```python
from build123d import *

# Parameters (mm, degrees)
F1_DEPTH = 101.6
F2_W     = 62.831107527
F2_H     = 56.3771557063
F3_DEPTH = 36.068
F4_W     = 26.6572609544
F4_H     = 13.4982671589
F4_H_2   = 14.6736167371
F5_DEPTH = 108.712
F6_R     = 7.0273260197
F6_R_2   = 6.9955111579
F6_R_3   = 6.6555032816
F6_R_4   = 6.7798018692
F7_DEPTH = 174.752


with BuildPart() as f1:
    # F0 (on Front) → F1 (new body)
    with BuildSketch(Plane.XZ):
        Polygon((-7.4572972953, 38.0593240261), (-75.9830623865, 38.0593240261), (-75.9830623865, -18.1280076504), (0, -18.1280076504), (0, -31.7951962352), (76.0644078255, -31.7951962352), align=None)
    extrude(amount=F1_DEPTH)

    # F2 (on face) → F3 (cut)
    with BuildSketch(Plane.XZ.offset(101.6)):
        with Locations((59.3193974346, -3.606618382)):
            Rectangle(F2_W, F2_H)
    extrude(amount=-F3_DEPTH, mode=Mode.SUBTRACT)

    # F4 (on face) → F5 (cut)
    with BuildSketch(Plane(origin=(-75.9830623865, 0, 0), x_dir=(0, -1, 0), z_dir=(-1, 0, 0))):
        with Locations((50.1333586872, 31.3101904467)):
            Rectangle(F4_W, F4_H)
        with Locations((50.1333586872, 45.3961323947)):
            Rectangle(F4_W, F4_H_2)
    extrude(amount=-F5_DEPTH, mode=Mode.SUBTRACT)

    # F6 (on face) → F7 (cut)
    with BuildSketch(Plane(origin=(-75.9830623865, 0, 0), x_dir=(0, -1, 0), z_dir=(-1, 0, 0))):
        with Locations((51.6176335514, -6.4415424131)):
            Circle(F6_R)
        with Locations((51.6176335514, 13.1108649075)):
            Circle(F6_R_2)
        with Locations((17.7108142525, -6.4415424131)):
            Circle(F6_R_3)
        with Locations((17.7108142525, 15.2898039669)):
            Circle(F6_R_4)
    extrude(amount=-F7_DEPTH, mode=Mode.SUBTRACT)


solid = f1.part
```
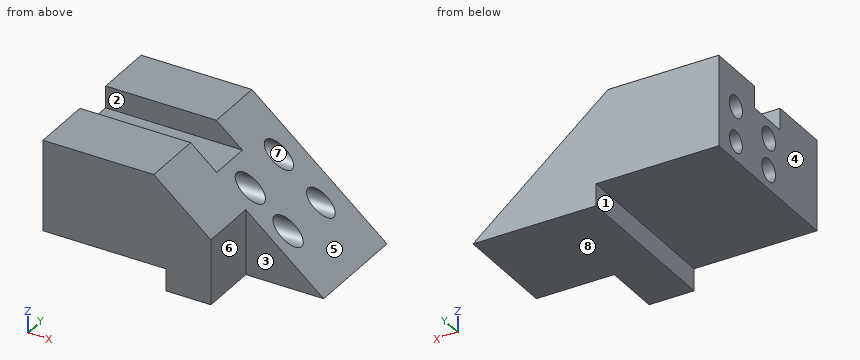
The listing builds one solid part. Answer for the finished solid, in the listing's coordinates (mm). Face numbers are marked on the shaded views. A direction names the side the tool comes from. Round coordinates to 2 decimals unless told otherwise and drop trailing zeros. Write each loop counter-clockwise with the first axis right and the second up, starting at its lowest first coordinate (ties: lowest second). Pieces come first, ordered by that corner, then holes. Notation, with made-up numbers: (89.5, 60) -> (115.5, 60) arc R30 cw to (115.5, 83) -> close; hole circle Ø8 at (-13.75, -14.5). An arc over 180 degrees is marked (long way). Answer as a JSON object with one key per item and string values. Group by question number.
Q1. Section B-B (z = 29.5) is taken. Write down the section's boundary in (x, y), plus the area to 3 significant figures.
Q2. Section D-D (z = -11.5) is taken. Write down the section's boundary in (x, y), plus the area to 3 significant figures.
Q3. Section A-A (x = -4) is taken. Write down the section's boundary in (y, z), plus the area to 3 significant figures.
Q4. Section C-C (y = -71) is taken. Write down the section's boundary in (x, z), plus the area to 3 significant figures.
Q5. Each of these flat-tipped pins is pushed along its axis until it touches: pin 1 Ø12.5 at (y, z) = (-51.62, -6.44) entering from -X; pin 2 Ø5 at (y, z) = (-77.5, -24) entering from -X; pin 3 Ø12 at (y, z) = (-15, 14) entering from +X; pin 4 Ø6 at (x, y) = (-34, -49.5) entering from +Z. Where does it stop, or does it pass through?
Q6. Which of the six approach directions +Z, -Z, +X, -X, +Y, -Y give full straight-line access (tool end or side, diameter ignored) to the marked faces 1, 2, 3, 4 and 5?
Q7. Straight lines are drawn through the part: line 1 along Z through (x, y) = (-57, -17); line 2 along Y through (x, z) = (12, 10); line 3 along Y through (x, z) = (-46, 15). For each, find the intervals that lie inside material, in ascending order.
Q8. Determine the mould class of the marked faces 6, 7 and 8 for opening direction Z: pulls with the +Z half, pulls with the -Z half, needs draft (parallel to the pull), parting line crosses it, or undercut.
Check values:
{
 "1": {"outline": "(-75.98, -101.6) -> (2.78, -101.6) -> (2.78, -63.46) -> (-75.98, -63.46) -> close; (-75.98, -36.8) -> (2.78, -36.8) -> (2.78, 0) -> (-75.98, 0) -> close", "area": "5,900 mm^2"},
 "2": {"outline": "(-75.98, -101.6) -> (27.9, -101.6) -> (27.9, -65.53) -> (51.8, -65.53) -> (51.8, -56.5) -> (-75.98, -56.5) -> close; (-75.98, -46.74) -> (51.8, -46.74) -> (51.8, -22.04) -> (-75.98, -22.04) -> close; (-75.98, -13.39) -> (51.8, -13.39) -> (51.8, 0) -> (-75.98, 0) -> close", "area": "9,770 mm^2"},
 "3": {"outline": "(-101.6, -18.13) -> (0, -18.13) -> (0, 35.17) -> (-36.8, 35.17) -> (-36.8, 24.56) -> (-63.46, 24.56) -> (-63.46, 35.17) -> (-101.6, 35.17) -> close; hole circle Ø14.05 at (-51.62, -6.44); hole circle Ø13.99 at (-51.62, 13.11); hole circle Ø13.56 at (-17.71, 15.29); hole circle Ø13.31 at (-17.71, -6.44)", "area": "4,540 mm^2"},
 "4": {"outline": "(-75.98, -18.13) -> (0, -18.13) -> (0, -31.8) -> (27.9, -31.8) -> (27.9, 8.48) -> (-7.46, 38.06) -> (-75.98, 38.06) -> close", "area": "5,700 mm^2"},
 "5": {"pin 1": "through", "pin 2": "x = 0", "pin 3": "x = 28.48", "pin 4": "z = 24.56"},
 "6": {"face 1": "-Z, -X, +Y, -Y", "face 2": "+Z, +X, -X", "face 3": "+Z, -Z, +X, -Y", "face 4": "+Z, -Z, -X, +Y, -Y", "face 5": "+Z, +X, +Y, -Y"},
 "7": {"line 1": "-18.13 to -13.06, 0.18 to 8.55, 22.03 to 38.06", "line 2": "-101.6 to -57.88, -45.35 to -21.95, -13.47 to 0", "line 3": "-101.6 to -58.35, -44.88 to -24.48, -10.94 to 0"},
 "8": {"face 6": "needs draft", "face 7": "undercut", "face 8": "pulls with the -Z half"}
}
